The listing builds one solid part. Answer for the finished solid, in the listing's coordinates (mm). A direction names the side the tool comes from. Round coordinates to 2 decimals unless told otherwise and drop trailing zeros. Order: outer loops, then holes, each group sorted by start corner. A loop starts at its lowest first (then second) coordinate and runs counter-clockwise, first axis right, second up. Notation, with made-up numbers: (-39, -15) -> (-7, -15) arc R25 ccw to (-7, 16) -> close; hole circle Ø1 at (64.25, -29). An arc over 180 degrees is marked (long way). Return JSON: item names as keys, results as strings. Group by question number.
(1) Each of these flat-tipped pins is pushed along its axis until it touches: pin 1 (1 mm diameter, centred on x = -25.5, z = -12, fed in from -Y); pin 2 (4 mm diameter, centred on x = -21, y = -12.5, fed in from +Z); pin 3 (6 mm diameter, centred on x = 2, y = -10, fed in from +Z). Where does it stop, or does it pass through?
(2) The part is cut by section C-C (x = 16.5). Determine the outline of the cut face in (y, z), plus the area to 3 significant figures.
(3) Which of the six approach directions +Z, -Z, +X, -X, +Y, -Y give full straight-line access (tool end or side, diameter ignored) to faces 5 (the face through (-25, -4.75, -12)), 6 (the face through (-36, -7.6, -11.5)), 7 (the face through (-6, -2, -6))?
(4) The part is cut by section A-A (x = 0). Determine the outline of the cut face in (y, z).
(5) Determine the mould class of faces 1 (the face through (-1.08, -14.51, -4.88)), 2 (the face through (-0.867, -0.986, -3.905)), 3 (the face through (0.77, -14.486, 6.958)), 4 (the face through (14.29, -9.78, -12.01)) for opening direction Z: +Z half, -Z half, draft (parallel to the pull), parting line (faces both ways), or undercut.
(6) The part is cut by section D-D (z = 0). Determine the outline of the cut face in (x, y).
(7) Consider line 1 (X direction, y = -7.75, z = -11.9); line 2 (Y direction, x = -24.5, z = -10); line 3 (Z direction, x = 16, y = -13). Determine where each line is inside the solid, lowest interval first. Write a range as [from, to].
(8) The part is cut by section B-B (z = -9.5). Determine the outline of the cut face in (x, y), plus the area to 3 significant figures.
from build123d import *

# Parameters (mm, degrees)
F0_R     = 5
F0_R_2   = 4
F1_DEPTH = 15.5
F2_W     = 11.5
F2_H     = 26.2481089791
F2_H_2   = 4
F3_DEPTH = 59.001
F4_R     = 3
F5_DEPTH = 2
F6_R     = 1
F7_R     = 2
F8_R     = 5
F8_R_2   = 4
F9_DEPTH = 2


# Not quite as in the source:
# - a feature names something its author has since deleted; it is built from what else it names


with BuildPart() as f1:
    # F0 (on Front) → F1 (new body)
    with BuildSketch(Plane.XZ):
        with BuildLine():
            Line((-36, -7), (-4.54e-08, -7))
            ThreePointArc((-4.54e-08, -7), (-6.871307732, -1.3360875914), (-2.6230483271, 6.4899628253))
            Line((-2.6230483271, 6.4899628253), (-36, -7))
        make_face()
        Polygon((23, -7), (-4.54e-08, -7), (-36, -7), (-36, -13), (23, -13), align=None)
        with BuildLine():
            ThreePointArc((3.8996539792, 5.8131487889), (6.1764705882, 3.2941176471), (7, 0))
            ThreePointArc((7, 0), (4.9497474522, -4.9497474844), (-4.54e-08, -7))
            Line((-4.54e-08, -7), (23, -7))
            Line((23, -7), (3.8996539792, 5.8131487889))
        make_face()
        with BuildLine():
            ThreePointArc((-4.54e-08, -7), (4.9497474522, -4.9497474844), (7, 0))
            ThreePointArc((7, 0), (6.1764705882, 3.2941176471), (3.8996539792, 5.8131487889))
            ThreePointArc((3.8996539792, 5.8131487889), (0.7224609385, 6.9626180559), (-2.6230483271, 6.4899628253))
            ThreePointArc((-2.6230483271, 6.4899628253), (-6.871307732, -1.3360875914), (-4.54e-08, -7))
        make_face()
        Circle(F0_R, mode=Mode.SUBTRACT)
        Circle(F0_R)
        Circle(F0_R_2, mode=Mode.SUBTRACT)
    extrude(amount=F1_DEPTH)

    # F2 (on face) → F3 (cut, through all)
    with BuildSketch(Plane.YZ.offset(23)):
        with Locations((-7.75, 6.1240544895)):
            Rectangle(F2_W, F2_H)
        with Locations((-7.75, -9)):
            Rectangle(F2_W, F2_H_2)
    extrude(amount=-F3_DEPTH, mode=Mode.SUBTRACT)

    # F4 (on face) → F5 (cut)
    with BuildSketch(Plane(origin=(0, 0, -13), x_dir=(1, 0, 0), z_dir=(0, 0, -1))):
        with BuildLine():
            ThreePointArc((-29, 4.75), (-26.8786796564, 5.6286796564), (-26, 7.75))
            ThreePointArc((-26, 7.75), (-26.8786796564, 9.8713203436), (-29, 10.75))
            ThreePointArc((-29, 10.75), (-32, 7.75), (-29, 4.75))
        make_face()
        with BuildLine():
            ThreePointArc((-29, 10.75), (-26.8786796564, 9.8713203436), (-26, 7.75))
            ThreePointArc((-26, 7.75), (-26.8786796564, 5.6286796564), (-29, 4.75))
            Line((-29, 4.75), (-20.5, 4.75))
            ThreePointArc((-20.5, 4.75), (-23.5, 7.75), (-20.5, 10.75))
            Line((-20.5, 10.75), (-29, 10.75))
        make_face()
        with BuildLine():
            ThreePointArc((-17.5, 7.75), (-18.3786796564, 9.8713203436), (-20.5, 10.75))
            ThreePointArc((-20.5, 10.75), (-23.5, 7.75), (-20.5, 4.75))
            ThreePointArc((-20.5, 4.75), (-18.3786796564, 5.6286796564), (-17.5, 7.75))
        make_face()
        with Locations((16.5, 7.75)):
            Circle(F4_R)
    extrude(amount=-F5_DEPTH, mode=Mode.SUBTRACT)

    # F6
    f6_edges = [f1.edges().sort_by_distance(p)[0] for p in [
        (-36, -14.5, -7),
        (-36, -1, -7),
        (23, -14.5, -7),
        (23, -1, -7),
    ]]
    fillet(f6_edges, radius=F6_R)

    # F7
    f7_edges = [f1.edges().sort_by_distance(p)[0] for p in [
        (-6.5, -15.5, -13),
        (-6.5, 0, -13),
    ]]
    fillet(f7_edges, radius=F7_R)

    # F8 (on face) → F9 (cut, through all)
    with BuildSketch(Plane.XZ.offset(15.5)):
        Circle(F8_R)
        Circle(F8_R_2, mode=Mode.SUBTRACT)
    extrude(amount=-F9_DEPTH, mode=Mode.SUBTRACT)


solid = f1.part
Answer below:
{
 "1": {"pin 1": "stops at y = -15.44", "pin 2": "stops at z = -0.24", "pin 3": "stops at z = -11"},
 "2": {"outline": "(-15.5, -11) arc R2 ccw to (-13.5, -13) -> (-10.75, -13) -> (-10.75, -11) -> (-13.5, -11) -> (-13.5, -2.64) -> (-15.5, -2.64) -> close; (-4.75, -13) -> (-2, -13) arc R2 ccw to (0, -11) -> (0, -2.64) -> (-2, -2.64) -> (-2, -11) -> (-4.75, -11) -> close", "area": "50.7 mm²"},
 "3": {"face 5": "+Z, -Z", "face 6": "+Z, -Z, -X, +Y, -Y", "face 7": "+Z, +X, -X"},
 "4": {"outline": "(-15.5, -11) arc R2 ccw to (-13.5, -13) -> (-2, -13) arc R2 ccw to (0, -11) -> (0, -4) -> (-2, -4) -> (-2, -11) -> (-13.5, -11) -> (-13.5, -5) -> (-15.5, -5) -> close; (-15.5, 5) -> (-13.5, 5) -> (-13.5, 7) -> (-15.5, 7) -> close; (-2, 4) -> (0, 4) -> (0, 7) -> (-2, 7) -> close"},
 "5": {"face 1": "undercut", "face 2": "undercut", "face 3": "+Z half", "face 4": "draft"},
 "6": {"outline": "(-18.68, -15.5) -> (-5, -15.5) -> (-5, -13.5) -> (-18.68, -13.5) -> close; (-18.68, -2) -> (-4, -2) -> (-4, 0) -> (-18.68, 0) -> close; (4, -2) -> (12.57, -2) -> (12.57, 0) -> (4, 0) -> close; (5, -15.5) -> (12.57, -15.5) -> (12.57, -13.5) -> (5, -13.5) -> close"},
 "7": {"line 1": "x = [-36, -32], [-17.5, 13.5], [19.5, 23]", "line 2": "y = [-15.5, -13.5], [-2, 0]", "line 3": "z = [-13, -11]"},
 "8": {"outline": "(-36, -15.5) -> (23, -15.5) -> (23, -13.5) -> (-36, -13.5) -> close; (-36, -2) -> (23, -2) -> (23, 0) -> (-36, 0) -> close", "area": "236 mm²"}
}
